```python
from build123d import *

# Parameters (mm, degrees)
SKETCH2_W           = 100
SKETCH2_H           = 80
SKETCH2_R           = 3
BOSS_EXTRUDE1_DEPTH = 10
SKETCH3_W           = 100
SKETCH3_H           = 10
BOSS_EXTRUDE2_DEPTH = 20
CUT_EXTRUDE1_REACH  = 82.336
SKETCH4_R           = 2.5


with BuildPart() as part:
    # Sketch2 → Boss-Extrude1 (new body)
    with BuildSketch(Plane.XY):
        with Locations((0, -2.079062729)):
            Rectangle(SKETCH2_W, SKETCH2_H)
        with Locations((27.5, 27.920937271)):
            Circle(SKETCH2_R, mode=Mode.SUBTRACT)
        with Locations((-27.5, 27.920937271)):
            Circle(SKETCH2_R, mode=Mode.SUBTRACT)
        with Locations(Location((-27.5, -32.079062729, 0), (0, 0, 180))):
            Circle(SKETCH2_R, mode=Mode.SUBTRACT)
        with Locations(Location((27.5, -32.079062729, 0), (0, 0, 180))):
            Circle(SKETCH2_R, mode=Mode.SUBTRACT)
    extrude(amount=BOSS_EXTRUDE1_DEPTH)

    # Sketch3 → Boss-Extrude2 (add)
    with BuildSketch(Plane.XZ.offset(42.079062729)):
        with Locations((0, 5)):
            Rectangle(SKETCH3_W, SKETCH3_H)
    extrude(amount=BOSS_EXTRUDE2_DEPTH)

    # Sketch4 → Cut-Extrude1 (cut, up to next)
    with BuildSketch(Plane.XY.offset(10), mode=Mode.PRIVATE) as cut_extrude1_sk1:
        with Locations((0, -57.079062729)):
            Circle(SKETCH4_R)
    cut_extrude1_tool1 = extrude(cut_extrude1_sk1.sketch, amount=-CUT_EXTRUDE1_REACH, mode=Mode.PRIVATE) & part.part
    # Sketch4 → Cut-Extrude1 (cut, up to next)
    with BuildSketch(Plane.XY.offset(10), mode=Mode.PRIVATE) as cut_extrude1_sk2:
        with Locations((-35, -57.079062729)):
            Circle(SKETCH4_R)
    cut_extrude1_tool2 = extrude(cut_extrude1_sk2.sketch, amount=-CUT_EXTRUDE1_REACH, mode=Mode.PRIVATE) & part.part
    # Sketch4 → Cut-Extrude1 (cut, up to next)
    with BuildSketch(Plane.XY.offset(10), mode=Mode.PRIVATE) as cut_extrude1_sk3:
        with Locations((35, -57.079062729)):
            Circle(SKETCH4_R)
    cut_extrude1_tool3 = extrude(cut_extrude1_sk3.sketch, amount=-CUT_EXTRUDE1_REACH, mode=Mode.PRIVATE) & part.part
    add(cut_extrude1_tool1.solids().sort_by_distance((0, -57.079063, 10))[0], mode=Mode.SUBTRACT)
    add(cut_extrude1_tool2.solids().sort_by_distance((-35, -57.079063, 10))[0], mode=Mode.SUBTRACT)
    add(cut_extrude1_tool3.solids().sort_by_distance((35, -57.079063, 10))[0], mode=Mode.SUBTRACT)


solid = part.part
```
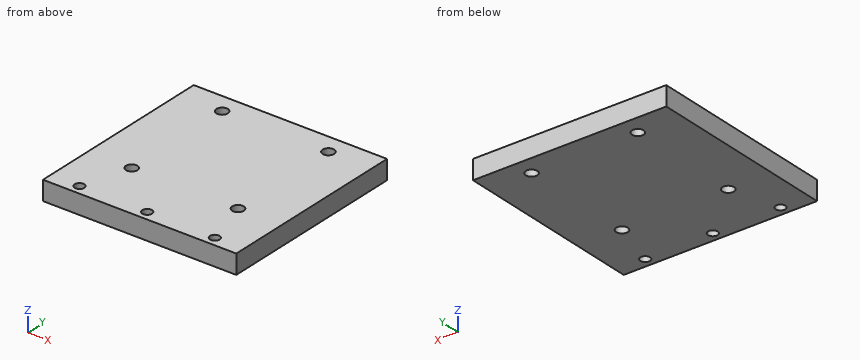
Model file for the job. Use its own axes, mm. Round coordinates to 2 decimals unless told otherwise and drop trailing zeros. Write each loop counter-clockwise with the first axis right and the second up, starting at its lowest first coordinate (ties: lowest second). Pieces come first, ordered by that corner, then holes. Notation, with made-up numbers: (11.25, 89.25) - (66.25, 89.25) arc R11 cw to (66.25, 106.25) - close; hole circle Ø1 at (84, 30.5). An arc over 180 degrees is marked (long way). Use CSV: the item, a comma, the result in double quotes. Start each with the question number.
Item 1: Band-saw the part on C-C (z = 6.25). Write the cut outline in (x, y).
Item 2: Pin check, flat tips, straight feed: P1, Ø8, axis at x = -35, y = -57.08, coming from the +Z side; P2, Ø5, axis at x = -27.5, y = -32.08, coming from the -Z side (3 decimals). Stop position of each tip, or through.
Item 3: Band-saw the part on A-A (x = 27.5). Write the cut outline in (y, z), and give its area (3 significant figures).
Item 4: Drill centre lines: L1, parallel to Y at x = -27.5, z = 8; L2, parallel to Y at x = -35, z = 7.5; L3, parallel to X at y = -30, z = 9.75. Where is each one in solid material? Low to high. Write a range as [from, to].
Item 5: Band-saw the part on B-B (x = 0). Write the cut outline in (y, z).
Item 6: Band-saw the part on D-D (x = -29). Write the cut outline in (y, z).
Checked values:
1,outline,"(-50, -62.08) - (50, -62.08) - (50, 37.92) - (-50, 37.92) - close; hole circle Ø5 at (-35, -57.08); hole circle Ø6 at (-27.5, -32.08); hole circle Ø6 at (-27.5, 27.92); hole circle Ø5 at (0, -57.08); hole circle Ø6 at (27.5, -32.08); hole circle Ø6 at (27.5, 27.92); hole circle Ø5 at (35, -57.08)"
2,P1,"stops at z = 10"
2,P2,"passes through"
3,outline,"(-62.08, 0) - (-35.08, 0) - (-35.08, 10) - (-62.08, 10) - close; (-29.08, 0) - (24.92, 0) - (24.92, 10) - (-29.08, 10) - close; (30.92, 0) - (37.92, 0) - (37.92, 10) - (30.92, 10) - close"
3,area,"880 mm²"
4,L1,"y = [-62.08, -35.08], [-29.08, 24.92], [30.92, 37.92]"
4,L2,"y = [-62.08, -59.58], [-54.58, 37.92]"
4,L3,"x = [-50, -29.66], [-25.34, 25.34], [29.66, 50]"
5,outline,"(-62.08, 0) - (-59.58, 0) - (-59.58, 10) - (-62.08, 10) - close; (-54.58, 0) - (37.92, 0) - (37.92, 10) - (-54.58, 10) - close"
6,outline,"(-62.08, 0) - (-34.68, 0) - (-34.68, 10) - (-62.08, 10) - close; (-29.48, 0) - (25.32, 0) - (25.32, 10) - (-29.48, 10) - close; (30.52, 0) - (37.92, 0) - (37.92, 10) - (30.52, 10) - close"
